Geometry check sheet. Reference: the model listing, model coordinates, mm. Face numbers are marked on the shaded views. Round coordinates to 2 decimals unless told otherwise and drop trailing zeros. Order: outer loops, then holes, each group sorted by start corner. A loop starts at its lowest first (then second) coordinate and runs counter-clockwise, first axis right, second up. Notation, with made-up numbers: (-17, 0.5) -> (-2, 0.5) arc R12 ccw to (-2, 9.5) -> close; hole circle Ø11 at (30.25, 6.5). An arc over 180 degrees is marked (long way). Use a Markdown table: item, result. Add a question column.
Item 1: Sectioned sample at A-A, the plane y = 0.95. State how many separate pieces and enclosed holes the cut face has, and give its area (3 significant figures).
Item 2: Sectioned sample at D-D, the plane z = 9. Record the cut outline in (x, y).
Item 3: Material ranges on probe 1 along X at (y, z) = (1.4, -0.5); probe 2 along X at (y, z) = (0.5, 0.5); probe 3 along Z at (x, y) = (3.5, 2.25), recorded low to high. Write a range as [from, to].
Item 4: Mould release check, pull along X, two halves, no side actions. Record for the marked faces 1 and 2: pulls with the +X half, pulls with the -X half, needs draft (parallel to the pull), parting line crosses it, or undercut.
Item 5: Sectioned sample at C-C, the plane x = 8. Record the cut outline in (y, z), and give its area (3 significant figures).
Item 6: Sectioned sample at B-B, the plane z = -9. Record the cut outline in (x, y), and give its area (3 significant figures).
Item 7: Gauge pin test, flat ends, axial feed: pin 1 Ø1.7 at (x, z) = (15, 7.5) entering from +Y; pin 2 Ø1.5 at (y, z) = (2, -15.5) entering from -X; pin 3 Ø1.1 at (y, z) = (2.5, -19) entering from +X; pin 4 Ø5 at (x, z) = (-12.5, -6.5) entering from +Y. Record the tip position at first contact, or that the pin passes through.
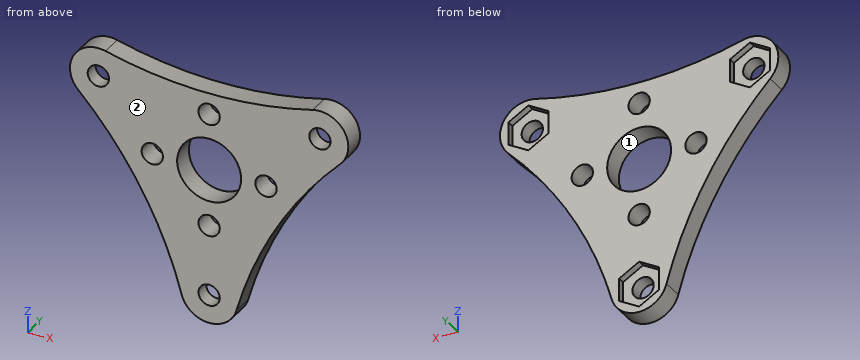
from build123d import *

# Parameters (mm, degrees)
SKETCH_1_R          = 1.5
SKETCH_1_R_2        = 4.5
EXTRUDE_1_DEPTH     = 3
CUT_EXTRUDE_1_DEPTH = 1


with BuildPart() as part:
    # 草图1 → 凸台-拉伸1 (new body)
    with BuildSketch(Plane(origin=(0, 0, 0), x_dir=(1, 0, 0), z_dir=(0, 1, 0))):
        with BuildLine():
            ThreePointArc((3.85699385, 19.059999265), (0, 22), (-3.85699385, 19.059999265))
            ThreePointArc((-3.85699385, 19.059999265), (-9.524981738, 5.499250771), (-18.434940485, -6.189744976))
            ThreePointArc((-18.434940485, -6.189744976), (-19.052558883, -11), (-14.577946635, -12.870254289))
            ThreePointArc((-14.577946635, -12.870254289), (0, -10.998501541), (14.577946635, -12.870254289))
            ThreePointArc((14.577946635, -12.870254289), (19.052558883, -11), (18.434940485, -6.189744976))
            ThreePointArc((18.434940485, -6.189744976), (9.524981738, 5.499250771), (3.85699385, 19.059999265))
        make_face()
        with Locations((8, 0)):
            Circle(SKETCH_1_R, mode=Mode.SUBTRACT)
        with Locations((0, -8)):
            Circle(SKETCH_1_R, mode=Mode.SUBTRACT)
        with Locations((-8, 0)):
            Circle(SKETCH_1_R, mode=Mode.SUBTRACT)
        with Locations((0, 8)):
            Circle(SKETCH_1_R, mode=Mode.SUBTRACT)
        with Locations((0, 18)):
            Circle(SKETCH_1_R, mode=Mode.SUBTRACT)
        with Locations((15.588457268, -9)):
            Circle(SKETCH_1_R, mode=Mode.SUBTRACT)
        with Locations((-15.588457268, -9)):
            Circle(SKETCH_1_R, mode=Mode.SUBTRACT)
        Circle(SKETCH_1_R_2, mode=Mode.SUBTRACT)
    extrude(amount=EXTRUDE_1_DEPTH)

    # 草图2 → 切除-拉伸1 (cut)
    with BuildSketch(Plane(origin=(0, 3, 0), x_dir=(1, 0, 0), z_dir=(0, 1, 0))):
        Polygon((0, 14.766838493), (2.8, 16.383419246), (2.8, 19.616580754), (0, 21.233161507), (-2.8, 19.616580754), (-2.8, 16.383419246), align=None)
        Polygon((12.788457268, -7.383419246), (12.788457268, -10.616580754), (15.588457268, -12.233161507), (18.388457268, -10.616580754), (18.388457268, -7.383419246), (15.588457268, -5.766838493), align=None)
        Polygon((-12.788457268, -7.383419246), (-15.588457268, -5.766838493), (-18.388457268, -7.383419246), (-18.388457268, -10.616580754), (-15.588457268, -12.233161507), (-12.788457268, -10.616580754), align=None)
    extrude(amount=-CUT_EXTRUDE_1_DEPTH, mode=Mode.SUBTRACT)


solid = part.part
Found:
| question | item | result |
|---|---|---|
| 1 | separate pieces | 1 |
| 1 | enclosed holes | 8 |
| 1 | area | 611 mm2 |
| 2 | outline | (-19.59, 0) -> (-17.09, 0) -> (-17.09, 2) -> (-18.39, 2) -> (-18.39, 3) -> (-19.59, 3) -> close; (-14.09, 0) -> (-1.12, 0) -> (-1.12, 3) -> (-12.79, 3) -> (-12.79, 2) -> (-14.09, 2) -> close; (1.12, 0) -> (14.09, 0) -> (14.09, 2) -> (12.79, 2) -> (12.79, 3) -> (1.12, 3) -> close; (17.09, 0) -> (19.59, 0) -> (19.59, 3) -> (18.39, 3) -> (18.39, 2) -> (17.09, 2) -> close |
| 3 | probe 1 | x = [-12.77, -9.41], [-6.59, -4.47], [4.47, 6.59], [9.41, 12.77] |
| 3 | probe 2 | x = [-13.51, -9.41], [-6.59, -4.47], [4.47, 6.59], [9.41, 13.51] |
| 3 | probe 3 | z = [-19.94, -2.83], [2.83, 11.1] |
| 4 | face 1 | undercut |
| 4 | face 2 | needs draft |
| 5 | outline | (0, -8.32) -> (3, -8.32) -> (3, -1.5) -> (0, -1.5) -> close; (0, 1.5) -> (3, 1.5) -> (3, 11.56) -> (0, 11.56) -> close |
| 5 | area | 50.6 mm2 |
| 6 | outline | (-7.66, 0) -> (-1.12, 0) -> (-1.12, 3) -> (-7.66, 3) -> close; (1.12, 0) -> (7.66, 0) -> (7.66, 3) -> (1.12, 3) -> close |
| 6 | area | 39.3 mm2 |
| 7 | pin 1 | stops at y = 2 |
| 7 | pin 2 | stops at x = -5.23 |
| 7 | pin 3 | stops at x = 4.03 |
| 7 | pin 4 | passes through |
